Geometry: final body of the model. Coordinates: model frame, mm. A direction names the side the tool comes from. Give positions to 0.01 mm unless a question says otherwise; leave off trailing zeros. Loops run counter-clockwise (first coordinate to the right, second up) from the corner with the lowest first, then second, coordinate; pieces in that order, holes last. Notation, with made-up numbers: (35, -13.75) -> (73, -13.75) arc R30 cw to (73, 9.25) -> close; hole circle Ø10 at (80.25, -6.5). An arc over 180 degrees is marked (long way). Answer in a Markdown table with one row per item. Add a question column.
1) Section query A-A (y = -64). Return the cut outline in (x, z).
2) Section query B-B (z = 0). Return the cut outline in (x, y).
3) Draft query along Y for faces 1 (the flat face through (0.077, -60.84, 37.203)), 2 (the cylindrical face through (0.921, -125.07, 90.986)), 3 (the flat face through (0, -125, 61)). Return one class per face: +Y half, -Y half, draft (parallel to the pull), parting line (faces both ways), or undercut.
4) Access query for faces 4 (the flat face through (7.5, -58, 32)), 5 (the flat face through (-7.5, -58, 32)), 6 (the flat face through (-5, -132, 25)), 7 (the flat face through (5.5, -60, 28)), 8 (the flat face through (-6.514, -59.16, 18.397)). Directions: +Z, -Z, +X, -X, +Y, -Y. A direction counts if a zero-diameter tool reaches every point of the face in a straight line with its end or side. Return the directions, or none.
5) Section query D-D (x = 20.5). Return the cut outline in (y, z), plus the area to 3 significant figures.
6) Section query C-C (z = 64). Return the cut outline in (x, y), plus the area to 3 significant figures.
7) Line query: line 1 (Z direction, x = 0, y = -128); line 2 (Z direction, x = 0, y = 2); line 3 (X direction, y = -94, z = 45.5). Output: solid intervals per line, ascending. Write a range as from..to.
8) First-contact query: P1, Ø12, axis at y = -49, z = 12.5, coming from the +X side; P2, Ø2, axis at x = 3, y = -132.5, coming from the +Z side; P3, Ø3, axis at x = 1.5, z = 1, coming from the -Y side. Flat tips, straight axial feed; report the tip coordinate or a pass-through.
```python
from build123d import *

# Parameters (mm, degrees)
SKETCH_W     = 15
SKETCH_H     = 20
SKETCH_R     = 2.75
PAD_DEPTH    = 3
PAD001_DEPTH = 2
PAD002_DEPTH = 5.5
PAD003_DEPTH = 5
SKETCH004_R  = 28.3
POCKET_DEPTH = 5
PAD004_DEPTH = 3


with BuildPart() as part:
    # Sketch → Pad (new body)
    with BuildSketch(Plane.XZ):
        Rectangle(SKETCH_W, SKETCH_H)
        Circle(SKETCH_R, mode=Mode.SUBTRACT)
    extrude(amount=-PAD_DEPTH)

    # Sketch001 (on DatumPlane) → Pad001 (join)
    with BuildSketch(Plane.YZ.offset(7.5)):
        Polygon((0, -10), (-125, 50), (-125, 70), (0, 10), align=None)
    pad001 = extrude(amount=-PAD001_DEPTH)

    # Mirrored: Pad001 across YZ
    add(pad001.mirror(Plane.YZ))

    # Sketch002 → Pad002 (join, symmetric)
    with BuildSketch(Plane.YZ):
        Polygon((0, 10), (-125, 70), (-125, 68), (0, 8), align=None)
    extrude(amount=PAD002_DEPTH, both=True)

    # Sketch003 (on DatumPlane) → Pad003 (join, symmetric)
    with BuildSketch(Plane.XZ.offset(125)):
        with BuildLine():
            ThreePointArc((24.372074, 43.507087), (0, 91), (-24.372074, 43.507087))
            Line((-24.372074, 43.507087), (-7.5, 20))
            Line((-7.5, 20), (7.5, 20))
            Line((7.5, 20), (24.372074, 43.507087))
        make_face()
    extrude(amount=PAD003_DEPTH, both=True)

    # Sketch004 (on DatumPlane) → Pocket (cut)
    with BuildSketch(Plane.XZ.offset(125)):
        with Locations((0, 61)):
            Circle(SKETCH004_R)
    extrude(amount=POCKET_DEPTH, mode=Mode.SUBTRACT)

    # Sketch005 (on DatumPlane) → Pad004 (join, symmetric)
    with BuildSketch(Plane.XY.offset(28)):
        with BuildLine():
            ThreePointArc((0, -130), (-2.828427, -131.171573), (-4, -134))
            Line((-4, -134), (-5, -134))
            Line((-5, -134), (-10, -130))
            Line((-10, -130), (0, -130))
        make_face()
    pad004 = extrude(amount=PAD004_DEPTH, both=True)

    # Mirrored001: Pad004 across Sketch005 V_Axis
    add(pad004.mirror(Plane(origin=(0, 0, 28), x_dir=(0, 0, 1), z_dir=(1, 0, 0))))


solid = part.part
```
Evaluation:
| question | item | result |
|---|---|---|
| 1 | outline | (-7.5, 20.72) -> (-5.5, 20.72) -> (-5.5, 38.72) -> (5.5, 38.72) -> (5.5, 20.72) -> (7.5, 20.72) -> (7.5, 40.72) -> (-7.5, 40.72) -> close |
| 2 | outline | (-7.5, -20.83) -> (-5.5, -20.83) -> (-5.5, 0) -> (-2.75, 0) -> (-2.75, 3) -> (-7.5, 3) -> close; (2.75, 0) -> (5.5, 0) -> (5.5, -20.83) -> (7.5, -20.83) -> (7.5, 3) -> (2.75, 3) -> close |
| 3 | face 1 | undercut |
| 3 | face 2 | draft |
| 3 | face 3 | -Y half |
| 4 | face 4 | +Z, -Z, +X, +Y |
| 4 | face 5 | +Z, -Z, -X, +Y |
| 4 | face 6 | -Z, +X, -X, -Y |
| 4 | face 7 | -Z |
| 4 | face 8 | -Z, +X, -X |
| 5 | outline | (-130, 38.11) -> (-120, 38.11) -> (-120, 82.9) -> (-130, 82.9) -> (-130, 80.51) -> (-125, 80.51) -> (-125, 41.49) -> (-130, 41.49) -> close |
| 5 | area | 253 mm² |
| 6 | outline | (-29.85, -130) -> (-28.14, -130) -> (-28.14, -125) -> (28.14, -125) -> (28.14, -130) -> (29.85, -130) -> (29.85, -120) -> (7.5, -120) -> (7.5, -112.5) -> (-7.5, -112.5) -> (-7.5, -120) -> (-29.85, -120) -> close; hole (-5.5, -120) -> (5.5, -120) -> (5.5, -116.67) -> (-5.5, -116.67) -> close |
| 6 | area | 391 mm² |
| 7 | line 1 | 20..32.7, 89.3..91 |
| 7 | line 2 | -10..-2.75, 2.75..10 |
| 7 | line 3 | -7.5..-5.5, 5.5..7.5 |
| 8 | P1 | x = 7.5 |
| 8 | P2 | z = 31 |
| 8 | P3 | y = 0 |
